Verification items for the finished model (mm, model axes). A direction names the side the tool comes from. Give positions to 0.01 mm unless a question says otherwise; leave off trailing zeros. Order: outer loops, then holes, each group sorted by start corner. A loop starts at its lowest first (then second) coordinate and runs counter-clockwise, first axis right, second up. Notation, with made-up numbers: (21, -9.5) - (28, -9.5) arc R28 cw to (28, 17.5) - close; hole circle Ø4 at (-33.75, 13). An arc over 180 degrees is marked (long way). Answer as a JSON object with one key per item and string values.
```python
from build123d import *

# Parameters (mm, degrees)
F0_W          = 132.08
F0_H          = 111.76
F1_DEPTH      = 30.48
F3_DEPTH      = 25.4
F5_DEPTH      = 39.37
F5_DEPTH_BACK = 39.37
F7_DEPTH      = 127
F7_DEPTH_BACK = 127
F8_W          = 70.1737586008
F8_H          = 10.16
F9_DEPTH      = 124.52238
F10_W         = 219.0220057964
F10_H         = 191.3975924253
F11_DEPTH     = 40.60273


with BuildPart() as f1:
    # F0 (on Top) → F1 (new body)
    with BuildSketch(Plane.XY):
        Rectangle(F0_W, F0_H)
    extrude(amount=F1_DEPTH)

    # F2 (on face) → F3 (cut)
    with BuildSketch(Plane.XY.offset(30.48)):
        Polygon((55.88, 32.512), (-4.064, 32.512), (-4.064, 26.67), (-5.334, 26.67), (-5.334, 20.828), (-4.064, 20.828), (-4.064, -20.828), (-5.334, -20.828), (-5.334, -26.67), (-4.064, -26.67), (-4.064, -32.512), (55.88, -32.512), (55.88, -20.066), (61.0470063984, -20.066), (61.0470063984, 20.066), (55.88, 20.066), align=None)
    extrude(amount=-F3_DEPTH, mode=Mode.SUBTRACT)

    # F4 (on Front) → F5 (cut, two sides)
    with BuildSketch(Plane.XZ) as f5_sk:
        with BuildLine():
            Line((-56.7663048146, 9.8806022625), (-49.9083048146, 9.8806022625))
            ThreePointArc((-49.9083048146, 9.8806022625), (-34.1603048146, 1.9206995202), (-18.4123048146, 9.8806022625))
            Line((-18.4123048146, 9.8806022625), (-11.5543048146, 16.7386022625))
            Line((-11.5543048146, 16.7386022625), (-11.5543048146, 37.6269482076))
            Line((-11.5543048146, 37.6269482076), (-56.7663048146, 37.6269482076))
            Line((-56.7663048146, 37.6269482076), (-56.7663048146, 9.8806022625))
        make_face()
    extrude(amount=F5_DEPTH, mode=Mode.SUBTRACT)
    extrude(f5_sk.sketch, amount=-F5_DEPTH_BACK, mode=Mode.SUBTRACT)

    # F6 (on Front) → F7 (cut, two sides)
    with BuildSketch(Plane.XZ) as f7_sk:
        with BuildLine():
            Line((-38.3278677172, 31.1981041294), (-38.3278677172, 21.9360575249))
            ThreePointArc((-38.3278677172, 21.9360575249), (-34.4349396554, 17.2967755581), (-29.9718115766, 21.3904675121))
            Line((-29.9718115766, 21.3904675121), (-29.9718115766, 21.5672736871))
            Line((-29.9718115766, 21.5672736871), (-29.9718115766, 31.1981041294))
            Line((-29.9718115766, 31.1981041294), (-38.3278677172, 31.1981041294))
        make_face()
        with BuildLine():
            Line((-29.9718115766, 21.5672736871), (-29.9718115766, 21.3904675121))
            ThreePointArc((-29.9718115766, 21.3904675121), (-29.9708791052, 21.4788705996), (-29.9718115766, 21.5672736871))
        make_face()
    extrude(amount=-F7_DEPTH, mode=Mode.SUBTRACT)
    extrude(f7_sk.sketch, amount=F7_DEPTH_BACK, mode=Mode.SUBTRACT)

    # F8 (on face) → F9 (cut)
    with BuildSketch(Plane.XZ.offset(55.88)):
        with Locations((30.9531206996, 25.4)):
            Rectangle(F8_W, F8_H)
    extrude(amount=-F9_DEPTH, mode=Mode.SUBTRACT)

    # F10 (on face) → F11 (cut)
    with BuildSketch(Plane.XY.offset(30.48)):
        with Locations((0.9173303843, -3.9965510368)):
            Rectangle(F10_W, F10_H)
        Polygon((-66.04, -45.72), (-66.04, 45.72), (-46.482, 45.72), (-46.482, 60.96), (-21.082, 60.96), (-21.082, 45.72), (0, 45.72), (0, 38.862), (67.551702261, 38.862), (67.551702261, -38.862), (0, -38.862), (0, -45.72), (-21.082, -45.72), (-21.082, -60.96), (-46.482, -60.96), (-46.482, -45.72), align=None, mode=Mode.SUBTRACT)
    extrude(amount=-F11_DEPTH, mode=Mode.SUBTRACT)


solid = f1.part
```
(1) Section check C-C (x = 27.5). Record the cut outline in (y, z).
Computed values:
{"outline": "(-38.86, 0) - (38.86, 0) - (38.86, 20.32) - (32.51, 20.32) - (32.51, 5.08) - (-32.51, 5.08) - (-32.51, 20.32) - (-38.86, 20.32) - close"}
(2) Gauge pin test, flat ends, axial feed: pin 1 Ø19.5 at (x, y) = (32.5, 14) entering from +Z; pin 2 Ø5 at (y, z) = (-8, 25) entering from +X; pin 3 Ø8 at (x, z) = (44, 17) entering from -Y. Record the tip position at first contact, or that the pin passes through.
Computed values:
{"pin 1": "stops at z = 5.08", "pin 2": "stops at x = -4.13", "pin 3": "stops at y = -38.86"}
(3) Release check for a two-part mould opening along X. For faces 6 (the flat face through (25, -32.512, 13)), 7 (the flat face through (-46.482, -51, 15)), 8 (the flat face through (-11, 45.72, 15)) record: pulls with the +X half, pulls with the -X half, needs draft (parallel to the pull), parting line crosses it, or undercut.
Computed values:
{"face 6": "undercut", "face 7": "pulls with the -X half", "face 8": "needs draft"}
(4) Material ranges on line 1 along X through (y, z) = (33, 28); line 2 along X through (y, z) = (-43.5, 25); line 3 along Y through (x, z) = (19.5, 10.5), recorded low to high. Write a range as [from, to].
Computed values:
{"line 1": "x = [-66.04, -56.77], [-11.55, -4.13]", "line 2": "x = [-66.04, -38.33], [-29.97, -4.13]", "line 3": "y = [-38.86, -32.51], [32.51, 38.86]"}
(5) Section check B-B (y = -12). Record the cut outline in (x, z), then the cut area to 3 significant figures.
Computed values:
{"outline": "(-66.04, 0) - (66.04, 0) - (66.04, 20.32) - (61.05, 20.32) - (61.05, 5.08) - (-4.06, 5.08) - (-4.06, 20.32) - (-4.13, 20.32) - (-4.13, 30.48) - (-11.55, 30.48) - (-11.55, 16.74) - (-18.41, 9.88) arc R19.56 cw to (-49.91, 9.88) - (-56.77, 9.88) - (-56.77, 30.48) - (-66.04, 30.48) - close", "area": "1,240 mm²"}
(6) Access from +Z, -Z, +X, -X, +Y, -Y to the whole of each face (thin tool, end or side, straight path). Record for faces 1 (the flat face through (-4.134, -36, 25)), 2 (the flat face through (-56, 45.72, 15)), 3 (the flat face through (33, 38.862, 10)), 4 (the flat face through (33, -38.862, 10)), 5 (the cylindrical face through (-34.417, 0.551, 1.922)).
Computed values:
{"face 1": "+Z, +X, +Y, -Y", "face 2": "+Z, -Z, -X, +Y", "face 3": "+Z, -Z, +X, +Y", "face 4": "+Z, -Z, +X, -Y", "face 5": "+Z"}
(7) Section check D-D (y = 43). Record the cut outline in (x, z).
Computed values:
{"outline": "(-66.04, 0) - (0, 0) - (0, 20.32) - (-4.13, 20.32) - (-4.13, 30.48) - (-29.97, 30.48) - (-29.97, 21.57) arc R4.19 cw (long way) to (-38.33, 21.94) - (-38.33, 30.48) - (-66.04, 30.48) - close"}
